Geometry check sheet. Reference: drawing and pictorial views, mm from the part's lowest x, y, z. A direction names the side the tool comes from. Coordinates: 2 decimals unless noted, no trailing zeros. Loops run counter-clockwise (first coordinate to the right, second up) from the corner with the lowest first, then second, coordinate; pieces in that order, holes last. Notation, with made-up numbers: (48, -20) - (107, -20) arc R24 cw to (107, 4) - close; hole circle Ø3 at (52.25, 81). An arc over 180 degrees is marked (long way). One line per item, written item: value.
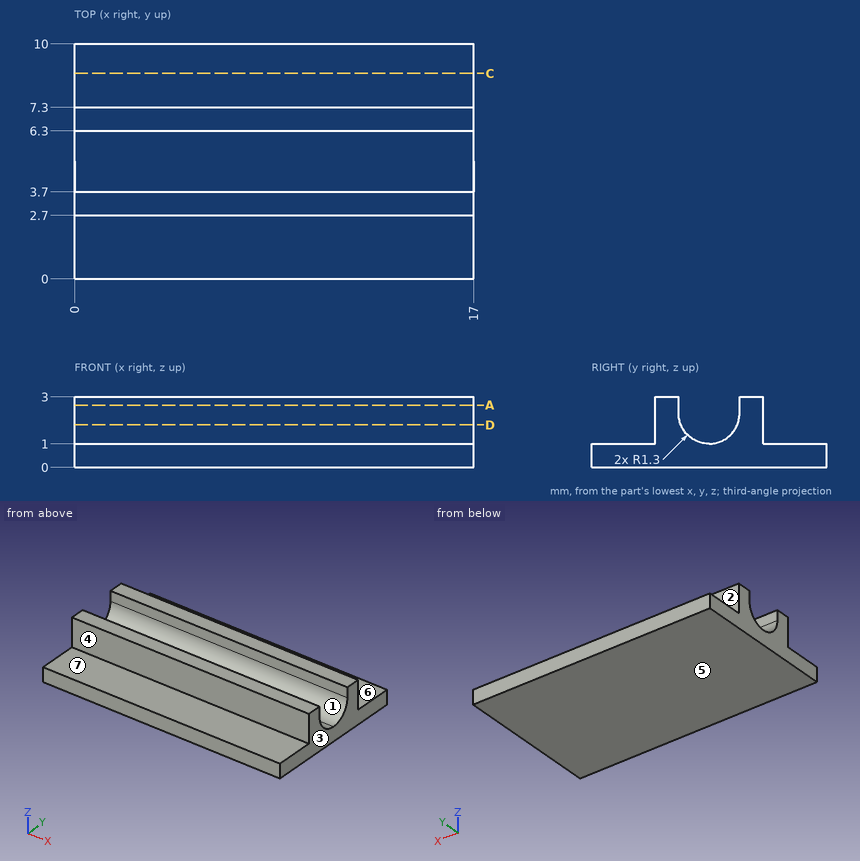
(1) Material ranges on probe 1 along Y at (x, z) = (0.5, 2.55); probe 2 along Z at (x, y) = (3.75, 7.5); probe 3 along Z at (x, y) = (8, 6), recorded low to high. Write a range as from..to.
Reply:
probe 1: 2.7..3.7, 6.3..7.3
probe 2: 0..1
probe 3: 0..1.47
(2) Access from +Z, -Z, +X, -X, +Y, -Y to the whole of each face (thin tool, end or side, straight path). Record for the marked faces 5, 6 and 7.
Reply:
face 5: -Z, +X, -X, +Y, -Y
face 6: +Z, +X, -X, +Y
face 7: +Z, +X, -X, -Y
(3) Cross-section at A-A on z = 2.65. Record the cut outline in (x, y), and give its area (3 significant figures).
Reply:
outline: (0, 2.7) - (17, 2.7) - (17, 3.7) - (0, 3.7) - close; (0, 6.3) - (17, 6.3) - (17, 7.3) - (0, 7.3) - close
area: 34.0 mm2
(4) Go/stop test with flat-tipped pins: pin 1 Ø1 at (x, z) = (4.5, 2) entering from +Y; pin 2 Ø1 at (x, z) = (8, 2) entering from -Y; pin 3 Ø2 at (x, y) = (6.5, 8.5) entering from +Z. Record where each tip stops, or that it passes through.
Reply:
pin 1: y = 7.3
pin 2: y = 2.7
pin 3: z = 1
(5) Cross-section at D-D on z = 1.8. Record the cut outline in (x, y), and give its area (3 significant figures).
Reply:
outline: (0, 2.7) - (17, 2.7) - (17, 3.8) - (0, 3.8) - close; (0, 6.2) - (17, 6.2) - (17, 7.3) - (0, 7.3) - close
area: 37.4 mm2
(6) Cross-section at C-C on y = 8.75. Record the cut outline in (x, z), and give its area (3 significant figures).
Reply:
outline: (0, 0) - (17, 0) - (17, 1) - (0, 1) - close
area: 17.0 mm2
(7) Release check for a two-part mould opening along Y. For the marked faces 1, 2, 3 and 4 record: pulls with the +Y half, pulls with the -Y half, needs draft (parallel to the pull), parting line crosses it, or undercut.
Reply:
face 1: undercut
face 2: pulls with the +Y half
face 3: needs draft
face 4: pulls with the -Y half
